from build123d import *

# Parameters (mm, degrees)
SKETCH1_R           = 30.5
SKETCH1_R_2         = 29
BOSS_EXTRUDE1_DEPTH = 15
SKETCH2_R           = 30.5
SKETCH2_R_2         = 27.5
BOSS_EXTRUDE2_DEPTH = 2
SKETCH3_R           = 30.5
SKETCH3_R_2         = 29
BOSS_EXTRUDE3_DEPTH = 15
BOSS_EXTRUDE4_DEPTH = 2
SKETCH5_R           = 1.6
CUT_EXTRUDE1_DEPTH  = 40


with BuildPart() as part:
    # Sketch1 → Boss-Extrude1 (new body)
    with BuildSketch(Plane(origin=(0, 0, 0), x_dir=(1, 0, 0), z_dir=(0, 1, 0))):
        with Locations(Location((0, 0, 0), (0, 0, 270))):
            Circle(SKETCH1_R)
        with Locations(Location((0, 0, 0), (0, 0, 270))):
            Circle(SKETCH1_R_2, mode=Mode.SUBTRACT)
    extrude(amount=BOSS_EXTRUDE1_DEPTH)

    # Sketch2 → Boss-Extrude2 (add)
    with BuildSketch(Plane(origin=(0, 15, 0), x_dir=(1, 0, 0), z_dir=(0, 1, 0))):
        with Locations(Location((0, 0, 0), (0, 0, 270))):
            Circle(SKETCH2_R)
        with Locations(Location((0, 0, 0), (0, 0, 270))):
            Circle(SKETCH2_R_2, mode=Mode.SUBTRACT)
    extrude(amount=BOSS_EXTRUDE2_DEPTH)

    # Sketch3 → Boss-Extrude3 (add)
    with BuildSketch(Plane(origin=(0, 17, 0), x_dir=(1, 0, 0), z_dir=(0, 1, 0))):
        with Locations(Location((0, 0, 0), (0, 0, 270))):
            Circle(SKETCH3_R)
        with Locations(Location((0, 0, 0), (0, 0, 270))):
            Circle(SKETCH3_R_2, mode=Mode.SUBTRACT)
    extrude(amount=BOSS_EXTRUDE3_DEPTH)

    # Sketch4 → Boss-Extrude4 (add)
    with BuildSketch(Plane(origin=(0, 26.5, 0), x_dir=(1, 0, 0), z_dir=(0, 1, 0))):
        with BuildLine():
            ThreePointArc((-32.429444444, -4.858900164), (-30.570387885, -5.892011652), (-29.503666667, -7.731988956))
            ThreePointArc((-29.503666667, -7.731988956), (-30.249891184, -3.897958868), (-30.5, 0))
            ThreePointArc((-30.5, 0), (-30.249891184, 3.897958868), (-29.503666667, 7.731988956))
            ThreePointArc((-29.503666667, 7.731988956), (-30.570387885, 5.892011652), (-32.429444444, 4.858900164))
            ThreePointArc((-32.429444444, 4.858900164), (-36.25, 0), (-32.429444444, -4.858900164))
        make_face()
    boss_extrude4 = extrude(amount=BOSS_EXTRUDE4_DEPTH)

    # Sketch5 → Cut-Extrude1 (cut)
    with BuildSketch(Plane(origin=(0, 32, 0), x_dir=(1, 0, 0), z_dir=(0, 1, 0))):
        with Locations(Location((-31.25, 0, 0), (0, 0, 299.256813925))):
            Circle(SKETCH5_R)
    cut_extrude1 = extrude(amount=-CUT_EXTRUDE1_DEPTH, mode=Mode.SUBTRACT)

    # Mirror1: Boss-Extrude4, Cut-Extrude1 across plane
    add(boss_extrude4.mirror(Plane(origin=(0, 0, 0), x_dir=(0, 0, 1), z_dir=(1, 0, 0))))
    add(cut_extrude1.mirror(Plane(origin=(0, 0, 0), x_dir=(0, 0, 1), z_dir=(1, 0, 0))), mode=Mode.SUBTRACT)


solid = part.part
Part model, mm, in its own coordinate system. A direction names the side the tool comes from. Coordinates: 2 decimals unless noted, no trailing zeros. Loops run counter-clockwise (first coordinate to the right, second up) from the corner with the lowest first, then second, coordinate; pieces in that order, holes last. Notation, with made-up numbers: M 10.25,-29 L 60.25,-29 A19 cw 60.25,0 Z; hole C 52.25,34 d8. An arc over 180 degrees is marked long. Use a Markdown table: item, result. Add a question column.
Q1. Cut at A-A (x = 0). Write the cut outline in (y, z).
Q2. Pin check, flat tips, straight feed: P1, Ø10, axis at x = 19, z = 13, coming from the -Y side; P2, Ø12, axis at x = 28.5, y = 20, coming from the -Z side; P3, Ø5, axis at x = 31.25, z = 0, coming from the -Y side; P4, Ø12, axis at x = 11.5, y = 8, coming from the +Z side. Stop position of each tip, or through.
Q3. Which spindle directions (+Z, -Z, +X, -X, +Y, -Y) get a long thin tool onto all of the face, cutting with end or side? Do faces 4 (the flat face through (22, 15, 17)), 5 (the cylindrical face through (-36.25, 27.49, -0.09)), 6 (the flat face through (22, 17, 17)). Say none if no direction does.
Q4. Cut at D-D (z = 0). Write the cut outline in (x, y).
Q5. Probe L1, parallel to X at y = 10.5, z = 0; L2, parallel to X at y = 16, z = 0; L3, parallel to Y at x = 28, z = -3.5. List the from-to ranges inside material, lowest first.
Q6. Mould opens along Z. For faces 1 (the cylindrical face through (-30.55, 27.49, -5.91)), 2 (the cylindrical face through (-11.107, 7.395, 26.789)), 3 (the flat face through (-34, 28.5, 0)) say: +Z half, -Z half, draft (parallel to the pull), parting line (faces both ways), or undercut.
Q7. Cut at C-C (z = -20.5). Write the cut outline in (x, y), and give its area (3 significant figures).
Worked out:
| question | item | result |
|---|---|---|
| 1 | outline | M 0,-30.5 L 32,-30.5 L 32,-29 L 17,-29 L 17,-27.5 L 15,-27.5 L 15,-29 L 0,-29 Z; M 0,29 L 15,29 L 15,27.5 L 17,27.5 L 17,29 L 32,29 L 32,30.5 L 0,30.5 Z |
| 2 | P1 | stops at y = 15 |
| 2 | P2 | stops at z = -20.59 |
| 2 | P3 | stops at y = 0 |
| 2 | P4 | stops at z = 30 |
| 3 | face 4 | -Y |
| 3 | face 5 | -X, +Y, -Y |
| 3 | face 6 | +Y |
| 4 | outline | M -36.25,26.5 L -32.85,26.5 L -32.85,28.5 L -36.25,28.5 Z; M -29.65,0 L -29,0 L -29,15 L -27.5,15 L -27.5,17 L -29,17 L -29,32 L -29.65,32 Z; M 27.5,15 L 29,15 L 29,0 L 29.65,0 L 29.65,32 L 29,32 L 29,17 L 27.5,17 Z; M 32.85,26.5 L 36.25,26.5 L 36.25,28.5 L 32.85,28.5 Z |
| 5 | L1 | x = -29.65 to -29, 29 to 29.65 |
| 5 | L2 | x = -29.65 to -27.5, 27.5 to 29.65 |
| 5 | L3 | y = 15 to 17 |
| 6 | face 1 | -Z half |
| 6 | face 2 | undercut |
| 6 | face 3 | draft |
| 7 | outline | M -22.58,0 L -20.51,0 L -20.51,15 L -18.33,15 L -18.33,17 L -20.51,17 L -20.51,32 L -22.58,32 Z; M 18.33,15 L 20.51,15 L 20.51,0 L 22.58,0 L 22.58,32 L 20.51,32 L 20.51,17 L 18.33,17 Z |
| 7 | area | 141 mm2 |
